```python
from build123d import *

# Parameters (mm, degrees)
F0_W     = 50
F0_H     = 50
F1_DEPTH = 10
F4_DEPTH = 150
F5_W     = 18.2143148659
F5_H     = 17.1242148423
F6_DEPTH = 15
F8_D     = 3
F8_DEPTH = 50
F8_TIP   = 0.9012909285


with BuildPart() as f1:
    # F0 (on Front) → F1 (new body)
    with BuildSketch(Plane.XZ):
        with Locations((-32.8713305295, -26.3395220041)):
            Rectangle(F0_W, F0_H)
    extrude(amount=F1_DEPTH)

    # F3 (on face) → F4 (join)
    with BuildSketch(Plane.XZ.offset(10)):
        with BuildLine():
            ThreePointArc((-27.7835671151, -31.4272854184), (-26.1262573971, -28.9793373511), (-25.5436490476, -26.0811150074))
            ThreePointArc((-25.5436490476, -26.0811150074), (-36.0539043669, -19.2117363664), (-38.1272124911, -31.5954039658))
            Line((-38.1272124911, -31.5954039658), (-32.8713305295, -26.3395220041))
            Line((-32.8713305295, -26.3395220041), (-27.7835671151, -31.4272854184))
        make_face()
        with BuildLine():
            ThreePointArc((-38.1272124911, -31.5954039658), (-36.0539043669, -19.2117363664), (-25.5436490476, -26.0811150074))
            ThreePointArc((-25.5436490476, -26.0811150074), (-26.1262573971, -28.9793373511), (-27.7835671151, -31.4272854184))
            Line((-27.7835671151, -31.4272854184), (-24.2479633333, -34.9628892003))
            ThreePointArc((-24.2479633333, -34.9628892003), (-21.5068368486, -30.8927638189), (-20.5436490476, -26.0811150074))
            ThreePointArc((-20.5436490476, -26.0811150074), (-37.9675398455, -14.5917590894), (-41.6644969533, -35.1326884279))
            Line((-41.6644969533, -35.1326884279), (-38.1272124911, -31.5954039658))
        make_face()
        with BuildLine():
            Line((-32.8713305295, -26.3395220041), (-38.1272124911, -31.5954039658))
            ThreePointArc((-38.1272124911, -31.5954039658), (-32.921765268, -33.580124565), (-27.7835671151, -31.4272854184))
            Line((-27.7835671151, -31.4272854184), (-32.8713305295, -26.3395220041))
        make_face()
        with BuildLine():
            ThreePointArc((-27.7835671151, -31.4272854184), (-32.921765268, -33.580124565), (-38.1272124911, -31.5954039658))
            Line((-38.1272124911, -31.5954039658), (-41.6644969533, -35.1326884279))
            ThreePointArc((-41.6644969533, -35.1326884279), (-32.9217884335, -38.5805209929), (-24.2479633333, -34.9628892003))
            Line((-24.2479633333, -34.9628892003), (-27.7835671151, -31.4272854184))
        make_face()
    extrude(amount=F4_DEPTH)

    # F5 (on face) → F6 (join)
    with BuildSketch(Plane.XZ.offset(160)):
        with Locations((-33.0436490476, -26.0811150074)):
            Rectangle(F5_W, F5_H)
    extrude(amount=F6_DEPTH)

    # F8
    with Locations(Plane.YZ.offset(-23.9364916147)):
        with Locations((-167.5, -26.0811150074)):
            Hole(F8_D / 2, depth=F8_DEPTH)
            with Locations((0, 0, -(F8_DEPTH + F8_TIP / 2))):  # 118° drill point
                Cone(0, F8_D / 2, F8_TIP, mode=Mode.SUBTRACT)


solid = f1.part
```
The listing builds one solid part. Answer for the finished solid, in the listing's coordinates (mm). A direction names the side the tool comes from. Give positions to 0.01 mm unless a question says otherwise; leave off trailing zeros. Order: outer loops, then holes, each group sorted by start corner. A loop starts at its lowest first (then second) coordinate and runs counter-clockwise, first axis right, second up.
1) For faces 4 (the face through (-33, -160, -36)), 5 (the face through (-23, -160, -26)), 6 (the face through (-43, -160, -26)), 7 (the face through (-33, -160, -16)), determine the directions among +Z, -Z, +X, -X, +Y, -Y from which every point of the face is accessible in a straight line to the end or side of a thin tool.
Reported:
face 4: -Z, +X, -X, -Y
face 5: +Z, -Z, +X, -Y
face 6: +Z, -Z, -X, -Y
face 7: +Z, +X, -X, -Y
2) Determine the mould class of faces 1 (the face through (-33, -5, -51.34)), 2 (the face through (-33.171, -168.886, -26.656)), 3 (the face through (-42.151, -165.7, -26.2)) for opening direction Z: pulls with the +Z half, pulls with the -Z half, needs draft (parallel to the pull), parting line crosses it, or undercut.
Reported:
face 1: pulls with the -Z half
face 2: undercut
face 3: needs draft
3) Find section D-D on z = -31. Write down the section's boundary in (x, y).
Reported:
outline: (-57.87, -10) - (-44.54, -10) - (-44.54, -160) - (-42.15, -160) - (-42.15, -175) - (-23.94, -175) - (-23.94, -160) - (-21.55, -160) - (-21.55, -10) - (-7.87, -10) - (-7.87, 0) - (-57.87, 0) - close
4) Find section B-B on z = -5.5. Write down the section's boundary in (x, y).
Reported:
outline: (-57.87, -10) - (-7.87, -10) - (-7.87, 0) - (-57.87, 0) - close
5) Find section C-C on x = -15. Write down the section's boundary in (y, z), then the cut area to 3 significant figures.
Reported:
outline: (-10, -51.34) - (0, -51.34) - (0, -1.34) - (-10, -1.34) - close
area: 500 mm2
6) Given P1, Ø12, axis at y = -165.5, z = -30, coming from the +X side; P2, Ø2, axis at x = -19, z = -18.5, coming from the -Y side; P3, Ø7.5, axis at x = -31, y = -169, coming from the +Z side, each flat-ended and moving along its own axis, determine where each tip first touches the part or whether it passes through.
Reported:
P1: stops at x = -20.64
P2: stops at y = -10
P3: stops at z = -17.52
7) Find section A-A on y = -117.5. Write down the section's boundary in (x, z).
Reported:
outline: circle Ø25 at (-33.04, -26.08)
8) Consider line 1 along Z through (x, y) = (-27.25, -167.5); line 2 along X through (y, z) = (-51.5, -26); line 3 along Y through (x, z) = (-24, -15). Determine where each line is inside the solid, lowest interval first.
Reported:
line 1: z = -34.64 to -27.58, -24.58 to -17.52
line 2: x = -45.54 to -20.54
line 3: y = -10 to 0
